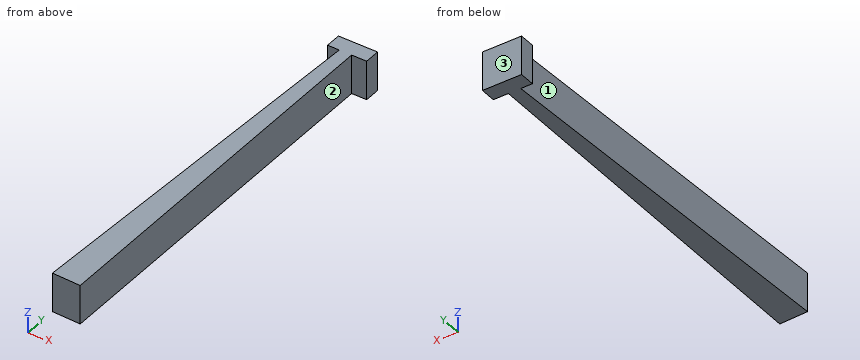
```python
from build123d import *

# Parameters (mm, degrees)
BOSS_EXTRUDE1_DEPTH = 50


with BuildPart() as part:
    # Sketch1 → Boss-Extrude1 (new body)
    with BuildSketch(Plane.XY):
        Polygon((15.05518629, 93.72842378), (9.296047762, 93.72842378), (-0.786164341, 93.72842378), (-21.44867742, -404.758474142), (15.05518629, -406.27157622), align=None)
        Polygon((-0.786164341, 93.72842378), (9.296047762, 93.72842378), (15.05518629, 93.72842378), (34.296047762, 93.72842378), (34.296047762, 113.72842378), (-15.703952238, 113.72842378), (-15.703952238, 93.72842378), align=None)
    extrude(amount=BOSS_EXTRUDE1_DEPTH)


solid = part.part
```
For this review, take the finished solid that the model builds, in its own axes (mm). Face numbers are marked on the shaded views. Coordinates: 2 decimals unless noted, no trailing zeros. Write each loop counter-clockwise with the first axis right and the second up, starting at its lowest first coordinate (ties: lowest second). Pieces come first, ordered by that corner, then holes. Notation, with made-up numbers: (73.5, 16) - (86.5, 16) arc R28 ccw to (86.5, 55) - close; hole circle Ø7 at (55.5, -21). An arc over 180 degrees is marked (long way). Answer in a Markdown table with one row per item. Add a question column.
Q1. For probe 1 along Y at (x, z) = (22, 31); probe 2 along Y at (x, z) = (15, 8); probe 3 along X at (y, z) = (-370.5, 31.5), list the stretches that pass through material, from the lowest coordinate up.
Q2. Draft analysis for pull direction Y (two halves, no side actions). For the marked faces 1, 2 and 3, state which applies: +Y half, -Y half, draft (parallel to the pull), parting line (faces both ways), or undercut.
Q3. We need section B-B, the plane y = -63. State the section outline as (x, z) points, and give its area (3 significant figures).
Q4. We need section C-C, the plane y = -123.5. State the section outline as (x, z) points, and give its area (3 significant figures).
Q5. We need section A-A, the plane z = 37.5. State the section outline as (x, y) points, and give its area (3 significant figures).
Q6. For P1, Ø16, axis at y = 100.5, z = 22.5, coming from the -X side; P2, Ø21, axis at x = 29.5, z = 33, coming from the -Y side; P3, Ø4.5, axis at x = -11, z = 27.5, coming from the -Y side, all flat-tipped, find the tip position at first contact; note any pin that passes through.
Answer list:
| question | item | result |
|---|---|---|
| 1 | probe 1 | y = 93.73 to 113.73 |
| 1 | probe 2 | y = -406.27 to 113.73 |
| 1 | probe 3 | x = -20.03 to 15.06 |
| 2 | face 1 | undercut |
| 2 | face 2 | draft |
| 2 | face 3 | +Y half |
| 3 | outline | (-7.28, 0) - (15.06, 0) - (15.06, 50) - (-7.28, 50) - close |
| 3 | area | 1,120 mm2 |
| 4 | outline | (-9.79, 0) - (15.06, 0) - (15.06, 50) - (-9.79, 50) - close |
| 4 | area | 1,240 mm2 |
| 5 | outline | (-21.45, -404.76) - (15.06, -406.27) - (15.06, 93.73) - (34.3, 93.73) - (34.3, 113.73) - (-15.7, 113.73) - (-15.7, 93.73) - (-0.79, 93.73) - close |
| 5 | area | 14,100 mm2 |
| 6 | P1 | stops at x = -15.7 |
| 6 | P2 | stops at y = 93.73 |
| 6 | P3 | stops at y = -405.28 |
